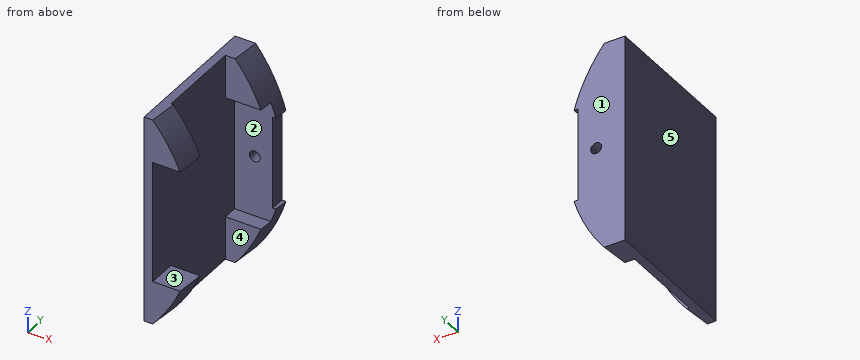
from build123d import *

# Parameters (mm, degrees)
CUT_EXTRUDE1_DEPTH      = 57.15
CUT_EXTRUDE2_DEPTH      = 57.15
CUT_EXTRUDE3_DEPTH      = 106.018320578
CUT_EXTRUDE3_DEPTH_BACK = 106.018320578
SKETCH7_W               = 43.8822002
SKETCH7_H               = 38.1
SKETCH8_R               = 2.38125
CUT_EXTRUDE4_DEPTH      = 57.15


with BuildPart() as part:
    # Sketch1 for Loft1 → Loft1 section 0
    with BuildSketch(Plane(origin=(0, 0, 0), x_dir=(1, 0, 0), z_dir=(0, 1, 0))):
        with BuildLine():
            Line((47.55805847, 45.81966963), (47.55805847, -45.81966963))
            Line((47.55805847, -45.81966963), (51.36805847, -45.81966963))
            # circular arc as an exact rational Bezier (weights 1, cos(half-angle), 1)
            Bezier((51.36805847, -45.81966963), (92.238634224, 0), (51.36805847, 45.81966963), weights=[1, 0.746259966, 1])
            Line((51.36805847, 45.81966963), (47.55805847, 45.81966963))
        make_face()
    # Sketch2 for Loft1 → Loft1 section 1
    with BuildSketch(Plane(origin=(0, 63.5, 0), x_dir=(1, 0, 0), z_dir=(0, 1, 0))):
        with BuildLine():
            Line((47.55805847, 45.81966963), (47.55805847, -45.81966963))
            Line((47.55805847, -45.81966963), (56.698115303, -45.81966963))
            Bezier((56.698115303, -45.81966963), (93.726544094, 0), (56.698115303, 45.81966963), weights=[1, 0.777773263, 1])
            Line((56.698115303, 45.81966963), (47.55805847, 45.81966963))
        make_face()
    loft()

    # Sketch5 → Cut-Extrude1 (cut)
    with BuildSketch(Plane.XZ):
        with BuildLine():
            ThreePointArc((63.415332088, -26.76966963), (68.834, 0), (63.415332088, 26.76966963))
            Line((63.415332088, 26.76966963), (51.36805847, 26.76966963))
            Line((51.36805847, 26.76966963), (51.36805847, -26.76966963))
            Line((51.36805847, -26.76966963), (63.415332088, -26.76966963))
        make_face()
        with BuildLine():
            Line((102.991666241, 26.76966963), (63.415332088, 26.76966963))
            ThreePointArc((63.415332088, 26.76966963), (68.834, 0), (63.415332088, -26.76966963))
            Line((63.415332088, -26.76966963), (102.991666241, -26.76966963))
            Line((102.991666241, -26.76966963), (102.991666241, 26.76966963))
        make_face()
    extrude(amount=-CUT_EXTRUDE1_DEPTH, mode=Mode.SUBTRACT)

    # Sketch6 → Cut-Extrude2 (cut)
    with BuildSketch(Plane(origin=(0, 63.5, 0), x_dir=(1, 0, 0), z_dir=(0, 1, 0))):
        with BuildLine():
            Line((103.737826736, 20.41966963), (69.979679166, 20.41966963))
            add(Edge.make_bspline(
                [(69.979679166, -20.419669631), (75.938021828, 0), (69.979679166, 20.419669631)],
                knots=[0.297886949, 0.297886949, 0.297886949, 0.702113051, 0.702113051, 0.702113051], degree=2, weights=[0.907042416, 0.870730847, 0.907042416]))
            Line((69.979679166, -20.41966963), (103.737826736, -20.41966963))
            Line((103.737826736, -20.41966963), (103.737826736, 20.41966963))
        make_face()
        with BuildLine():
            add(Edge.make_bspline(
                [(69.979679166, -20.419669631), (75.938021828, 0), (69.979679166, 20.419669631)],
                knots=[0.297886949, 0.297886949, 0.297886949, 0.702113051, 0.702113051, 0.702113051], degree=2, weights=[0.907042416, 0.870730847, 0.907042416]))
            Line((69.979679166, 20.41966963), (68.152482199, 20.41966963))
            Line((68.152482199, 20.41966963), (68.152482199, -20.41966963))
            Line((68.152482199, -20.41966963), (69.979679166, -20.41966963))
        make_face()
    extrude(amount=-CUT_EXTRUDE2_DEPTH, mode=Mode.SUBTRACT)

    # Sketch7 → Cut-Extrude3 (cut, two sides: drawn at the far end of the back side and taken through both)
    with BuildSketch(Plane.XY.offset(-CUT_EXTRUDE3_DEPTH_BACK)):
        with Locations((73.30915857, 31.75)):
            Rectangle(SKETCH7_W, SKETCH7_H)
    extrude(amount=CUT_EXTRUDE3_DEPTH + CUT_EXTRUDE3_DEPTH_BACK, mode=Mode.SUBTRACT)

    # Sketch8 → Cut-Extrude4 (cut)
    with BuildSketch(Plane.XZ.offset(-57.15)):
        with Locations(Location((60.25805847, -0.02733037, 0), (0, 0, 270))):
            Circle(SKETCH8_R)
    extrude(amount=-CUT_EXTRUDE4_DEPTH, mode=Mode.SUBTRACT)


solid = part.part
Verification items for the finished model (mm, model axes). Face numbers are marked on the shaded views. A direction names the side the tool comes from. Coordinates: 2 decimals unless noted, no trailing zeros. Write each loop counter-clockwise with the first axis right and the second up, starting at its lowest first coordinate (ties: lowest second). Pieces come first, ordered by that corner, then holes. Notation, with made-up numbers: M 71,1 L 108,1 A33 cw 108,30 Z; hole C 28,7.25 d7. An arc over 180 degrees is marked long. Use a Markdown table: item, result.
Q1. Sectioned sample at A-A, the plane z = 0. Record the boundary of the cut face in (x, y).
Reply:
| item | result |
|---|---|
| outline | M 47.56,0 L 51.37,0 L 51.37,57.15 L 57.88,57.15 L 57.88,63.5 L 47.56,63.5 Z; M 62.64,57.15 L 68.15,57.15 L 68.15,63.5 L 62.64,63.5 Z |
Q2. Sectioned sample at B-B, the plane z = -10. Record the boundary of the cut face in (x, y).
Reply:
| item | result |
|---|---|
| outline | M 47.56,0 L 51.37,0 L 51.37,57.15 L 68.15,57.15 L 68.15,63.5 L 47.56,63.5 Z |
Q3. Draft check along Z on the marked faces 1 and 2. Enter one of: +Z half, -Z half, draft (parallel to the pull), parting line (faces both ways), or undercut.
Reply:
| item | result |
|---|---|
| face 1 | draft |
| face 2 | undercut |
Q4. Go/stop test with flat-tipped pins: P1, Ø1.9, axis at x = 62.5, y = 53.5, coming from the +Z side; P2, Ø3, axis at y = 61.5, z = 4, coming from the +X side; P3, Ø4, axis at x = 54.5, y = 8, coming from the -Z side. Record where each tip stops, or that it passes through.
Reply:
| item | result |
|---|---|
| P1 | stops at z = 37.84 |
| P2 | stops at x = 68.15 |
| P3 | stops at z = -45.3 |
Q5. Thickness scan on line 1 (Z direction, x = 51.5, y = 51); line 2 (Y direction, x = 64.25, z = -6.5); line 3 (X direction, y = 40, z = -19.5). Record the ranges inside material, lowest first.
Reply:
| item | result |
|---|---|
| line 1 | z = -45.82 to -26.77, 26.77 to 45.82 |
| line 2 | y = 57.15 to 63.5 |
| line 3 | x = 47.56 to 51.37 |
Q6. Set-up check for the marked faces 3, 4 and 5: record each of +Z, -Z, +X, -X, +Y, -Y from which the full face is reachable in a straight line by a thin tool's end or side.
Reply:
| item | result |
|---|---|
| face 3 | +X, -Y |
| face 4 | +Z, -Z, +X |
| face 5 | +Z, -Z, -X, +Y, -Y |
